Build history of the part. All positions in model axes, mm. A direction names the side the tool comes from. Coordinates: 2 decimals unless noted, no trailing zeros. Order: outer loops, then holes, each group sorted by start corner. A loop starts at its lowest first (then second) coordinate and runs counter-clockwise, first axis right, second up. Notation, with made-up numbers: M 59.25,-1.75 L 73.25,-1.75 A20 cw 73.25,20.25 Z; hole C 4,37.25 d7. An arc over 180 degrees is marked long. Write item = value, one per line. Start each with the question number.
Q1. Pin check, flat tips, straight feed: P1, Ø5, axis at x = 73.5, z = -13, coming from the +Y side; P2, Ø1.2, axis at x = 161.5, y = 6, coming from the -Z side; P3, Ø5.5, axis at y = 2, z = -6.5, coming from the +X side; P4, Ø6, axis at x = 68, z = -3, coming from the +Y side. Stop position of each tip, or through.
Q2. Drill centre lines: probe 1 along Z at (x, y) = (135.5, 15); probe 2 along X at (y, z) = (1.45, -10); probe 3 along Y at (x, z) = (119.5, 21.5). Where is each one in solid material? Low to high.
Q3. Pull direction X, two halves, no side cores. Call faces 4 (the face through (160, 23, 25)), 5 (the face through (66.095, 2.465, -10.867)), 6 (the face through (79, 3, 25)): released by +X, released by -X, zero draft, split by the parting line, or undercut.
Q4. Band-saw the part on B-B on x = 70. Write the cut outline in (y, z).
Q5. 3-axis set-ups, long thin cutter, end or side, ignore diameter. For faces 1 (the face through (78, 23, 0)), 2 (the face through (70, 2, -19)), 3 (the face through (65.9, 5, -10.9)): which of +Z, -Z, +X, -X, +Y, -Y reach the whole face in a straight line?
Q6. Band-saw the part on D-D on z = 4.5. Write the cut outline in (x, y), plus the area to 3 significant figures.
Q7. Band-saw the part on C-C on y = 10.5. Write the cut outline in (x, z).
Q8. Band-saw the part on A-A on z = 32. Write the cut outline in (x, y), plus the area to 3 significant figures.
```python
from build123d import *

# Parameters (mm, degrees)
SKETCH_1_W             = 160
SKETCH_1_H             = 50
EXTRUDE_1_DEPTH        = 3
EXTRUDE_1_2_DEPTH      = 40
EXTRUDE_1_2_DEPTH_BACK = 3
SKETCH_3_W             = 165
SKETCH_3_H             = 55
SKETCH_3_W_2           = 160
SKETCH_3_H_2           = 50
SKETCH_4_W             = 50
SKETCH_4_H             = 40
CUT_EXTRUDE_1_DEPTH    = 100
CHAMFER_1_SIZE         = 1
CHAMFER_2_SIZE         = 1
SKETCH_1_4_R           = 4
EXTRUDE_8_DEPTH        = 5
SKETCH_8_W             = 8.5
SKETCH_8_H             = 10
CUT_EXTRUDE_3_DEPTH    = 10


with BuildPart() as part:
    # Sketch 1 → Extrude 1 (new body)
    with BuildSketch(Plane(origin=(0, 0, 0), x_dir=(1, 0, 0), z_dir=(0, 1, 0))):
        with Locations((80, -25)):
            Rectangle(SKETCH_1_W, SKETCH_1_H)
    extrude(amount=EXTRUDE_1_DEPTH)



with BuildPart() as body_2:
    # Sketch 3 → Extrude 1 2 (new, two sides: drawn at the far end of the back side and taken through both)
    with BuildSketch(Plane(origin=(0, 3, 0), x_dir=(1, 0, 0), z_dir=(0, 1, 0)).offset(-EXTRUDE_1_2_DEPTH_BACK)):
        with Locations((80, -25)):
            Rectangle(SKETCH_3_W, SKETCH_3_H)
        with Locations((80, -25)):
            Rectangle(SKETCH_3_W_2, SKETCH_3_H_2, mode=Mode.SUBTRACT)
    extrude(amount=EXTRUDE_1_2_DEPTH + EXTRUDE_1_2_DEPTH_BACK)

    # Sketch 4 → Cut-Extrude 1 (cut)
    with BuildSketch(Plane.ZY.offset(2.5)):
        with Locations((25, 23)):
            Rectangle(SKETCH_4_W, SKETCH_4_H)
    extrude(amount=-CUT_EXTRUDE_1_DEPTH, mode=Mode.SUBTRACT)

    # Chamfer 1
    chamfer_1_edges = [body_2.edges().sort_by_distance(p)[0] for p in [
        (162.5, 0, 25),
        (80, 0, -2.5),
        (-2.5, 0, 25),
        (80, 0, 52.5),
    ]]
    chamfer(chamfer_1_edges, length=CHAMFER_1_SIZE)

    # Chamfer 2
    chamfer_2_edges = [body_2.edges().sort_by_distance(p)[0] for p in [
        (162.5, 22, -2.5),
        (162.5, 22, 52.5),
    ]]
    chamfer(chamfer_2_edges, length=CHAMFER_2_SIZE)


with BuildPart() as part_1:
    add(part.part)

    add(body_2.part)  # Extrude 8 merges body 2
    # Sketch 1_4 → Extrude 8 (add)
    with BuildSketch(Plane(origin=(0, 0, 0), x_dir=(1, 0, 0), z_dir=(0, 1, 0))):
        with BuildLine():
            Line((61, 10), (61, 0))
            Line((61, 0), (70, 0))
            Line((70, 0), (79, 0))
            Line((79, 0), (79, 10))
            ThreePointArc((79, 10), (70, 19), (61, 10))
        make_face()
        with Locations(Location((70, 10, 0), (0, 0, 270))):
            Circle(SKETCH_1_4_R, mode=Mode.SUBTRACT)
    extrude(amount=EXTRUDE_8_DEPTH)

    # Sketch 8 → Cut-Extrude 3 (cut)
    with BuildSketch(Plane(origin=(162.5, 0, 0), x_dir=(0, 0, -1), z_dir=(1, 0, 0))):
        with Locations((-20.75, 8)):
            Rectangle(SKETCH_8_W, SKETCH_8_H)
        with Locations((-29.25, 8)):
            Rectangle(SKETCH_8_W, SKETCH_8_H)
    extrude(amount=-CUT_EXTRUDE_3_DEPTH, mode=Mode.SUBTRACT)


solid = part_1.part
```
Recorded:
q1.P1 = 5
q1.P2 = -2.5
q1.P3 = 79
q1.P4 = 43
q2.probe_1 = -2.5 to 0, 50 to 52.5
q2.probe_2 = 61 to 66, 74 to 79
q2.probe_3 = 0 to 3
q3.face_4 = released by -X
q3.face_5 = undercut
q3.face_6 = zero draft
q4.outline = M 0,-19 L 5,-19 L 5,-14 L 0,-14 Z; M 0,-6 L 5,-6 L 5,-2.5 L 43,-2.5 L 43,0 L 3,0 L 3,50 L 43,50 L 43,52.5 L 1,52.5 L 0,51.5 Z
q5.face_1 = -X, +Y
q5.face_2 = -Z, +Y, -Y
q5.face_3 = -Z, +X, -X, +Y
q6.outline = M -2.5,1 L -1.5,0 L 161.5,0 L 162.5,1 L 162.5,43 L 160,43 L 160,3 L -2.5,3 Z
q6.area = 594 mm2
q7.outline = M -2.5,-2.5 L 161.5,-2.5 L 162.5,-1.5 L 162.5,16.5 L 160,16.5 L 160,0 L -2.5,0 Z; M -2.5,50 L 160,50 L 160,33.5 L 162.5,33.5 L 162.5,51.5 L 161.5,52.5 L -2.5,52.5 Z
q8.outline = M -2.5,1 L -1.5,0 L 161.5,0 L 162.5,1 L 162.5,3 L -2.5,3 Z; M 160,13 L 162.5,13 L 162.5,43 L 160,43 Z
q8.area = 569 mm2
